```python
from build123d import *

# Parameters (mm, degrees)
SKETCH006_W     = 86
SKETCH006_H     = 101
SKETCH006_R     = 1.7
PAD002_DEPTH    = 2
SKETCH007_W     = 18.5
SKETCH007_H     = 31
SKETCH007_W_2   = 39
SKETCH007_H_2   = 13
POCKET002_DEPTH = 5
SKETCH008_W     = 86
SKETCH008_H     = 101
SKETCH008_W_2   = 66
SKETCH008_H_2   = 81
PAD003_DEPTH    = 3
SKETCH009_R     = 1.7
POCKET003_DEPTH = 3
SKETCH010_W     = 86
SKETCH010_H     = 101
SKETCH010_W_2   = 66
SKETCH010_H_2   = 81
PAD004_DEPTH    = 2
SKETCH011_W     = 18.5
SKETCH011_H     = 31
POCKET004_DEPTH = 5
FILLET001_R     = 5
CHAMFER_SIZE    = 2
CHAMFER001_SIZE = 2


with BuildPart() as part:
    # Sketch006 → Pad002 (new body)
    with BuildSketch(Plane.XY):
        with Locations((103.313661, -0.74487)):
            Rectangle(SKETCH006_W, SKETCH006_H)
        with Locations((141.313661, 44.75513)):
            Circle(SKETCH006_R, mode=Mode.SUBTRACT)
        with Locations((141.313661, -46.24487)):
            Circle(SKETCH006_R, mode=Mode.SUBTRACT)
        with Locations((65.313661, -46.24487)):
            Circle(SKETCH006_R, mode=Mode.SUBTRACT)
        with Locations((65.313661, 44.75513)):
            Circle(SKETCH006_R, mode=Mode.SUBTRACT)
        with BuildLine():
            Line((93.013661, 0.95513), (80.013661, 0.95513))
            ThreePointArc((79.513661, 1.45513), (79.660108, 1.101576), (80.013661, 0.95513))
            Line((79.513661, 1.45513), (79.513661, 14.45513))
            ThreePointArc((80.013661, 14.95513), (79.660108, 14.808683), (79.513661, 14.45513))
            Line((80.013661, 14.95513), (93.013661, 14.95513))
            ThreePointArc((93.513661, 14.45513), (93.367214, 14.808683), (93.013661, 14.95513))
            Line((93.513661, 14.45513), (93.513661, 1.45513))
            ThreePointArc((93.013661, 0.95513), (93.367214, 1.101576), (93.513661, 1.45513))
        make_face(mode=Mode.SUBTRACT)
        with BuildLine():
            Line((112.063661, 0.95513), (99.063661, 0.95513))
            ThreePointArc((98.563661, 1.45513), (98.710108, 1.101576), (99.063661, 0.95513))
            Line((98.563661, 1.45513), (98.563661, 14.45513))
            ThreePointArc((99.063661, 14.95513), (98.710108, 14.808683), (98.563661, 14.45513))
            Line((99.063661, 14.95513), (112.063661, 14.95513))
            ThreePointArc((112.563661, 14.45513), (112.417214, 14.808683), (112.063661, 14.95513))
            Line((112.563661, 14.45513), (112.563661, 1.45513))
            ThreePointArc((112.063661, 0.95513), (112.417214, 1.101576), (112.563661, 1.45513))
        make_face(mode=Mode.SUBTRACT)
        with BuildLine():
            Line((131.113661, 0.95513), (118.113661, 0.95513))
            ThreePointArc((117.613661, 1.45513), (117.760108, 1.101576), (118.113661, 0.95513))
            Line((117.613661, 1.45513), (117.613661, 14.45513))
            ThreePointArc((118.113661, 14.95513), (117.760108, 14.808683), (117.613661, 14.45513))
            Line((118.113661, 14.95513), (131.113661, 14.95513))
            ThreePointArc((131.613661, 14.45513), (131.467214, 14.808683), (131.113661, 14.95513))
            Line((131.613661, 14.45513), (131.613661, 1.45513))
            ThreePointArc((131.113661, 0.95513), (131.467214, 1.101576), (131.613661, 1.45513))
        make_face(mode=Mode.SUBTRACT)
        with BuildLine():
            Line((93.013661, -18.09487), (80.013661, -18.09487))
            ThreePointArc((79.513661, -17.59487), (79.660108, -17.948424), (80.013661, -18.09487))
            Line((79.513661, -17.59487), (79.513661, -4.59487))
            ThreePointArc((80.013661, -4.09487), (79.660108, -4.241317), (79.513661, -4.59487))
            Line((80.013661, -4.09487), (93.013661, -4.09487))
            ThreePointArc((93.513661, -4.59487), (93.367214, -4.241317), (93.013661, -4.09487))
            Line((93.513661, -4.59487), (93.513661, -17.59487))
            ThreePointArc((93.013661, -18.09487), (93.367214, -17.948424), (93.513661, -17.59487))
        make_face(mode=Mode.SUBTRACT)
        with BuildLine():
            Line((112.063661, -18.09487), (99.063661, -18.09487))
            ThreePointArc((98.563661, -17.59487), (98.710108, -17.948424), (99.063661, -18.09487))
            Line((98.563661, -17.59487), (98.563661, -4.59487))
            ThreePointArc((99.063661, -4.09487), (98.710108, -4.241317), (98.563661, -4.59487))
            Line((99.063661, -4.09487), (112.063661, -4.09487))
            ThreePointArc((112.563661, -4.59487), (112.417214, -4.241317), (112.063661, -4.09487))
            Line((112.563661, -4.59487), (112.563661, -17.59487))
            ThreePointArc((112.063661, -18.09487), (112.417214, -17.948424), (112.563661, -17.59487))
        make_face(mode=Mode.SUBTRACT)
        with BuildLine():
            Line((131.113661, -18.09487), (118.113661, -18.09487))
            ThreePointArc((117.613661, -17.59487), (117.760108, -17.948424), (118.113661, -18.09487))
            Line((117.613661, -17.59487), (117.613661, -4.59487))
            ThreePointArc((118.113661, -4.09487), (117.760108, -4.241317), (117.613661, -4.59487))
            Line((118.113661, -4.09487), (131.113661, -4.09487))
            ThreePointArc((131.613661, -4.59487), (131.467214, -4.241317), (131.113661, -4.09487))
            Line((131.613661, -4.59487), (131.613661, -17.59487))
            ThreePointArc((131.113661, -18.09487), (131.467214, -17.948424), (131.613661, -17.59487))
        make_face(mode=Mode.SUBTRACT)
        with BuildLine():
            Line((93.013661, -37.14487), (80.013661, -37.14487))
            ThreePointArc((79.513661, -36.64487), (79.660108, -36.998424), (80.013661, -37.14487))
            Line((79.513661, -36.64487), (79.513661, -23.64487))
            ThreePointArc((80.013661, -23.14487), (79.660108, -23.291317), (79.513661, -23.64487))
            Line((80.013661, -23.14487), (93.013661, -23.14487))
            ThreePointArc((93.513661, -23.64487), (93.367214, -23.291317), (93.013661, -23.14487))
            Line((93.513661, -23.64487), (93.513661, -36.64487))
            ThreePointArc((93.013661, -37.14487), (93.367214, -36.998424), (93.513661, -36.64487))
        make_face(mode=Mode.SUBTRACT)
        with BuildLine():
            Line((112.063661, -37.14487), (99.063661, -37.14487))
            ThreePointArc((98.563661, -36.64487), (98.710108, -36.998424), (99.063661, -37.14487))
            Line((98.563661, -36.64487), (98.563661, -23.64487))
            ThreePointArc((99.063661, -23.14487), (98.710108, -23.291317), (98.563661, -23.64487))
            Line((99.063661, -23.14487), (112.063661, -23.14487))
            ThreePointArc((112.563661, -23.64487), (112.417214, -23.291317), (112.063661, -23.14487))
            Line((112.563661, -23.64487), (112.563661, -36.64487))
            ThreePointArc((112.063661, -37.14487), (112.417214, -36.998424), (112.563661, -36.64487))
        make_face(mode=Mode.SUBTRACT)
        with BuildLine():
            Line((131.113661, -37.14487), (118.113661, -37.14487))
            ThreePointArc((117.613661, -36.64487), (117.760108, -36.998424), (118.113661, -37.14487))
            Line((117.613661, -36.64487), (117.613661, -23.64487))
            ThreePointArc((118.113661, -23.14487), (117.760108, -23.291317), (117.613661, -23.64487))
            Line((118.113661, -23.14487), (131.113661, -23.14487))
            ThreePointArc((131.613661, -23.64487), (131.467214, -23.291317), (131.113661, -23.14487))
            Line((131.613661, -23.64487), (131.613661, -36.64487))
            ThreePointArc((131.113661, -37.14487), (131.467214, -36.998424), (131.613661, -36.64487))
        make_face(mode=Mode.SUBTRACT)
    extrude(amount=PAD002_DEPTH)

    # Sketch007 → Pocket002 (cut, symmetric)
    with BuildSketch(Plane.XY.offset(2)):
        with Locations((123.989661, 34.25513)):
            Rectangle(SKETCH007_W, SKETCH007_H)
        with Locations((90.429661, 27.99613)):
            Rectangle(SKETCH007_W_2, SKETCH007_H_2)
    extrude(amount=POCKET002_DEPTH, both=True, mode=Mode.SUBTRACT)

    # Sketch008 (on Face5 of Pocket002) → Pad003 (join)
    with BuildSketch(Plane.XY.offset(2)):
        with Locations((103.313661, -0.74487)):
            Rectangle(SKETCH008_W, SKETCH008_H)
        with Locations((103.313661, 0)):
            Rectangle(SKETCH008_W_2, SKETCH008_H_2, mode=Mode.SUBTRACT)
    extrude(amount=PAD003_DEPTH)

    # Sketch009 (on Face92 of Pad003) → Pocket003 (cut)
    with BuildSketch(Plane.XY.offset(5)):
        with Locations((65.313661, 44.75513)):
            Circle(SKETCH009_R)
        with Locations((141.313661, 44.75513)):
            Circle(SKETCH009_R)
        with Locations((141.313661, -46.24487)):
            Circle(SKETCH009_R)
        with Locations((65.313661, -46.24487)):
            Circle(SKETCH009_R)
    extrude(amount=-POCKET003_DEPTH, mode=Mode.SUBTRACT)

    # Sketch010 (on Face85 of Pocket003) → Pad004 (join)
    with BuildSketch(Plane.XY.offset(5)):
        with Locations((103.313661, -0.74487)):
            Rectangle(SKETCH010_W, SKETCH010_H)
        with Locations((103.313661, 0)):
            Rectangle(SKETCH010_W_2, SKETCH010_H_2, mode=Mode.SUBTRACT)
    extrude(amount=PAD004_DEPTH)

    # Sketch011 (on Face92 of Pad004) → Pocket004 (cut)
    with BuildSketch(Plane.XY.offset(7)):
        with Locations((123.989661, 34.25513)):
            Rectangle(SKETCH011_W, SKETCH011_H)
    extrude(amount=-POCKET004_DEPTH, mode=Mode.SUBTRACT)

    # Fillet001
    fillet001_edges = [part.edges().sort_by_distance(p)[0] for p in [
        (146.313661, -51.24487, 3.5),
        (60.313661, -51.24487, 3.5),
        (146.313661, 49.75513, 3.5),
        (60.313661, 49.75513, 3.5),
    ]]
    fillet(fillet001_edges, radius=FILLET001_R)

    # Chamfer
    chamfer_edges = [part.edges().sort_by_distance(p)[0] for p in [
        (103.313661, -40.5, 7),
        (136.313661, 0, 7),
        (70.313661, 0, 7),
        (92.526661, 40.5, 7),
    ]]
    chamfer(chamfer_edges, length=CHAMFER_SIZE)

    # Chamfer001
    chamfer001_edges = [part.edges().sort_by_distance(p)[0] for p in [
        (60.313661, -0.74487, 7),
        (103.313661, -51.24487, 7),
        (61.778127, -49.780404, 7),
        (144.849195, -49.780404, 7),
        (146.313661, -0.74487, 7),
        (144.849195, 48.290663, 7),
        (137.276661, 49.75513, 7),
        (61.778127, 48.290663, 7),
        (90.026661, 49.75513, 7),
    ]]
    chamfer(chamfer001_edges, length=CHAMFER001_SIZE)


solid = part.part
```
Source: CAD feature listing. Evaluate the final solid. Frame: model axes, mm. A direction names the side the tool comes from. Coordinates: 2 decimals unless noted, no trailing zeros. Order: outer loops, then holes, each group sorted by start corner. A loop starts at its lowest first (then second) coordinate and runs counter-clockwise, first axis right, second up. Notation, with made-up numbers: (11.5, 27.5) - (59.5, 27.5) arc R11 cw to (59.5, 45.5) - close; hole circle Ø11 at (61.25, -21). An arc over 180 degrees is marked (long way). One line per item, written item: value.
1) Cut plane D-D on x = 130. Output: boundary loops of the cut face in (y, z).
Computed values:
outline: (-51.24, 0) - (-37.14, 0) - (-37.14, 2) - (-40.5, 2) - (-40.5, 5) - (-42.5, 7) - (-49.24, 7) - (-51.24, 5) - close; (-23.14, 0) - (-18.09, 0) - (-18.09, 2) - (-23.14, 2) - close; (-4.09, 0) - (0.96, 0) - (0.96, 2) - (-4.09, 2) - close; (14.96, 0) - (18.76, 0) - (18.76, 2) - (14.96, 2) - close
2) Reachability of faces 1 (the face through (146.314, -1, 2)), 2 (the face through (124, 18.755, 1)), 3 (the face through (87, -37.145, 1)), 4 (the face through (63.965, -47.279, 2.535)), 5 (the face through (92, 40.5, 3)) from +Z, -Z, +X, -X, +Y, -Y: full face, straight path, thin tool, end or side. Return the list, or none.
Computed values:
face 1: +Z, -Z, +X, +Y, -Y
face 2: +Z, -Z, +Y
face 3: +Z, -Z
face 4: -Z
face 5: +Z
3) Cut plane C-C on x = 86. Output: boundary loops of the cut face in (y, z).
Computed values:
outline: (-51.24, 0) - (-37.14, 0) - (-37.14, 2) - (-40.5, 2) - (-40.5, 5) - (-42.5, 7) - (-49.24, 7) - (-51.24, 5) - close; (-23.14, 0) - (-18.09, 0) - (-18.09, 2) - (-23.14, 2) - close; (-4.09, 0) - (0.96, 0) - (0.96, 2) - (-4.09, 2) - close; (14.96, 0) - (21.5, 0) - (21.5, 2) - (14.96, 2) - close; (34.5, 0) - (49.76, 0) - (49.76, 5) - (47.76, 7) - (42.5, 7) - (40.5, 5) - (40.5, 2) - (34.5, 2) - close
4) Mould query, pull axis Y, two halves, no side actions, for faces 6 (the face through (62.603, 47.407, 6.208)), 7 (the face through (70.93, 28, 1)), 8 (the face through (103, 0, 0)), 9 (the face through (91.2, 41.5, 6)). Classes: released by +Y, released by -Y, zero draft, split by the parting line, or undercut.
Computed values:
face 6: released by +Y
face 7: undercut
face 8: zero draft
face 9: undercut
5) Ray query, line 1 (Y direction, x = 84, z = 1.25); line 2 (X direction, y = 12.5, z = 4.25); line 3 (X direction, y = 32.5, z = 1.5). Return the intervals inside material, ascending. Write a range as [from, to].
Computed values:
line 1: y = [-51.24, -37.14], [-23.14, -18.09], [-4.09, 0.96], [14.96, 21.5], [34.5, 49.76]
line 2: x = [60.31, 70.31], [136.31, 146.31]
line 3: x = [60.31, 70.93], [109.93, 114.74], [133.24, 146.31]
6) Contact query for flat-ended pins moving along their axis: pin 1 (8 mm diameter, centred on x = 90, y = 23.5, fed in from +Z); pin 2 (1 mm diameter, centred on x = 123.5, z = 1.5, fed in from +Y). Output: stop coordinate, or through.
Computed values:
pin 1: stops at z = 2
pin 2: stops at y = 18.76
7) Cut plane A-A on x = 97. Output: boundary loops of the cut face in (y, z).
Computed values:
outline: (-51.24, 0) - (21.5, 0) - (21.5, 2) - (-40.5, 2) - (-40.5, 5) - (-42.5, 7) - (-49.24, 7) - (-51.24, 5) - close; (34.5, 0) - (49.76, 0) - (49.76, 5) - (47.76, 7) - (42.5, 7) - (40.5, 5) - (40.5, 2) - (34.5, 2) - close
8) Cut plane B-B on y = 38.5. Output: boundary loops of the cut face in (x, z).
Computed values:
outline: (60.31, 0) - (114.74, 0) - (114.74, 2) - (70.31, 2) - (70.31, 5) - (68.31, 7) - (62.31, 7) - (60.31, 5) - close; (133.24, 0) - (146.31, 0) - (146.31, 5) - (144.31, 7) - (138.31, 7) - (136.31, 5) - (136.31, 2) - (133.24, 2) - close
